Check sheet for the modelled part. Datum: model origin and axes. Units: mm. Face numbers are marked on the shaded views. A direction names the side the tool comes from. Round coordinates to 2 decimals unless told otherwise and drop trailing zeros. Order: outer loops, then holes, each group sorted by start corner. A loop starts at its lowest first (then second) coordinate and runs counter-clockwise, first axis right, second up.
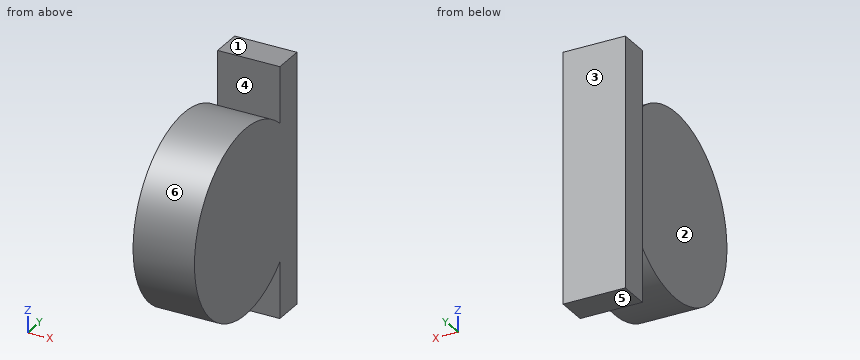
```python
from build123d import *

# Parameters (mm, degrees)
SKETCH3_W           = 25.753050404
SKETCH3_H           = 103.137359271
BOSS_EXTRUDE1_DEPTH = 12.7
SKETCH4_R           = 38.1
BOSS_EXTRUDE2_DEPTH = 25.4


with BuildPart() as part:
    # Sketch3 → Boss-Extrude1 (new body)
    with BuildSketch(Plane(origin=(0, 717.636591226, 0), x_dir=(-1, 0, 0), z_dir=(0, -1, 0))):
        with Locations((-511.2749233, -660.547915429)):
            Rectangle(SKETCH3_W, SKETCH3_H)
    extrude(amount=BOSS_EXTRUDE1_DEPTH)

    # Sketch4 → Boss-Extrude2 (add)
    with BuildSketch(Plane(origin=(524.151448502, 0, 0), x_dir=(0, 0, -1), z_dir=(1, 0, 0))):
        with Locations((-660.547915428, 679.536591226)):
            Circle(SKETCH4_R)
    extrude(amount=-BOSS_EXTRUDE2_DEPTH)


solid = part.part
```
Item 1: Go/stop test with flat-tipped pins: P1, Ø2, axis at x = 510.5, y = 696, coming from the -Z side; P2, Ø5, axis at x = 503, z = 619.5, coming from the -Y side; P3, Ø7.5, axis at x = 506.5, z = 681, coming from the -Y side. Record where each tip stops, or that it passes through.
Answer:
P1: stops at z = 625.73
P2: stops at y = 704.94
P3: stops at y = 645.29
Item 2: Sectioned sample at C-C (y = 659.5). Record the cut outline in (x, z), and give its area (3 significant figures).
Answer:
outline: (498.75, 628.14) - (524.15, 628.14) - (524.15, 692.95) - (498.75, 692.95) - close
area: 1,650 mm2
Item 3: Access from +Z, -Z, +X, -X, +Y, -Y to the whole of each face (thin tool, end or side, straight path). Record for the marked faces 1 and 2.
Answer:
face 1: +Z, +X, -X, +Y, -Y
face 2: +Z, -Z, -X, -Y
Item 4: Scan lines: line 1 along Y through (x, z) = (516.75, 626); line 2 along X through (y, z) = (681.5, 627.5); line 3 along Y through (x, z) = (505.25, 626.5). Record each from-to range of solid material in increasing order.
Answer:
line 1: y = 663.47 to 695.6, 704.94 to 717.64
line 2: x = 498.75 to 524.15
line 3: y = 662.44 to 696.63, 704.94 to 717.64
Item 5: Sectioned sample at B-B (z = 625). Record the cut outline in (x, y).
Answer:
outline: (498.4, 704.94) - (524.15, 704.94) - (524.15, 717.64) - (498.4, 717.64) - close; (498.75, 665.83) - (524.15, 665.83) - (524.15, 693.25) - (498.75, 693.25) - close
Item 6: Release check for a two-part mould opening along Y. For the marked faces 3, 4, 5 and 6 record: released by +Y, released by -Y, zero draft, split by the parting line, or undercut.
Answer:
face 3: released by +Y
face 4: undercut
face 5: zero draft
face 6: undercut
Item 7: Sectioned sample at A-A (z = 691.5). Record the cut outline in (x, y), and give its area (3 significant figures).
Answer:
outline: (498.4, 704.94) - (524.15, 704.94) - (524.15, 717.64) - (498.4, 717.64) - close; (498.75, 657.32) - (524.15, 657.32) - (524.15, 701.75) - (498.75, 701.75) - close
area: 1,460 mm2
Item 8: Sectioned sample at D-D (z = 645). Record the cut outline in (x, y), and give its area (3 significant figures).
Answer:
outline: (498.4, 704.94) - (498.75, 704.94) - (498.75, 644.75) - (524.15, 644.75) - (524.15, 717.64) - (498.4, 717.64) - close
area: 1,860 mm2
